Verification items for the finished model (mm, model axes). Coordinates: 2 decimals unless noted, no trailing zeros. Loops run counter-clockwise (first coordinate to the right, second up) from the corner with the lowest first, then second, coordinate; pieces in that order, holes last. Notation, with made-up numbers: (-21.5, 87.25) - (26.5, 87.25) arc R26 cw to (26.5, 125.25) - close; hole circle Ø9 at (-36.75, 78). An arc over 180 degrees is marked (long way). One line per item, written item: value. Start each with the question number.
(1) Draft check along X on faces 1 (the face through (3.95, 2.95, -6.72)), 2 (the face through (-7.794, 3, 0)), 3 (the face through (1.352, 2.958, 4.292)). Enter one of: +X half, -X half, draft (parallel to the pull), parting line (faces both ways), or undercut.
(2) Section check A-A (y = 1.9). Record the boundary of the cut face in (x, z), plus the area to 3 significant figures.
(3) Thickness scan on probe 1 along X at (y, z) = (1.65, 0); probe 2 along X at (y, z) = (4.2, -3); probe 3 along Z at (x, y) = (-0.25, 1). Record the ranges inside material, lowest first. Write a range as [from, to].
(4) Section check C-C (y = 5.4). Record the boundary of the cut face in (x, z), plus the area to 3 significant figures.
(5) Gauge pin test, flat ends, axial feed: P1, Ø7, axis at x = 0, z = 0, coming from the +Y side; P2, Ø2, axis at x = -0.5, y = 1.5, coming from the +Z side; P3, Ø2, axis at x = -3, z = 6, coming from the -Y side; P4, Ø2, axis at x = -1.5, y = 5, coming from the -Z side. Record the tip position at first contact, or that the pin passes through.
```python
from build123d import *

# Parameters (mm, degrees)
SKETCH3_R           = 4.5
BOSS_EXTRUDE2_DEPTH = 6
SKETCH4_OUTSIDE_W   = 42.5
SKETCH4_OUTSIDE_H   = 44.912
SKETCH4_OUTSIDE_R   = 7.768332991
CUT_EXTRUDE1_DEPTH  = 10
CUT_EXTRUDE1_DRAFT  = -45


with BuildPart() as part:
    # Sketch3 → Boss-Extrude2 (new body)
    with BuildSketch(Plane(origin=(0, 0, 0), x_dir=(1, 0, 0), z_dir=(0, 1, 0))):
        Polygon((0, -9), (7.794228634, -4.5), (7.794228634, 4.5), (0, 9), (-7.794228634, 4.5), (-7.794228634, -4.5), align=None)
        with Locations(Location((0, 0, 0), (0, 0, 270))):  # turned: the seam where the file's is
            Circle(SKETCH3_R, mode=Mode.SUBTRACT)
    extrude(amount=BOSS_EXTRUDE2_DEPTH)


with BuildPart() as cut_extrude1_tool:
    # Sketch4 outside → Cut-Extrude1 (with draft: the straight prism first)
    with BuildSketch(Plane(origin=(0, 6, 0), x_dir=(1, 0, 0), z_dir=(0, 1, 0))):
        Rectangle(SKETCH4_OUTSIDE_W, SKETCH4_OUTSIDE_H)
        Circle(SKETCH4_OUTSIDE_R, mode=Mode.SUBTRACT)
    extrude(amount=-CUT_EXTRUDE1_DEPTH)
    # Cut-Extrude1: the draft: its side faces are tilted about the plane it starts from
    cut_extrude1_sides = [cut_extrude1_tool.faces().sort_by_distance(p)[0] for p in [
        (0, 1, 22.456),
        (21.25, 1, 0),
        (0, 1, -22.456),
        (-21.25, 1, 0),
        (-7.768332991, 1, 0),
    ]]
    draft(cut_extrude1_sides, Plane(origin=(0, 6, 0), x_dir=(1, 0, 0), z_dir=(0, 1, 0)), CUT_EXTRUDE1_DRAFT)


with BuildPart() as part_1:
    add(part.part)

    # Cut-Extrude1: cut by cut_extrude1_tool
    add(cut_extrude1_tool.part, mode=Mode.SUBTRACT)


solid = part_1.part
```
Responses:
1. face 1: +X half
1. face 2: -X half
1. face 3: undercut
2. outline: (-7.79, -4.5) - (0, -9) - (7.79, -4.5) - (7.79, 4.5) - (0, 9) - (-7.79, 4.5) - close; hole circle Ø9 at (0, 0)
2. area: 147 mm²
3. probe 1: x = [-7.79, -4.5], [4.5, 7.79]
3. probe 2: x = [-7.79, -3.35], [3.35, 7.79]
3. probe 3: z = [-8.86, -4.49], [4.49, 8.86]
4. outline: (-7.79, -3.05) arc R8.37 ccw to (-6.54, -5.23) - (-1.26, -8.27) arc R8.37 ccw to (1.26, -8.27) - (6.54, -5.23) arc R8.37 ccw to (7.79, -3.05) - (7.79, 3.05) arc R8.37 ccw to (6.54, 5.23) - (1.26, 8.27) arc R8.37 ccw to (-1.26, 8.27) - (-6.54, 5.23) arc R8.37 ccw to (-7.79, 3.05) - close; hole circle Ø9 at (0, 0)
4. area: 142 mm²
5. P1: passes through
5. P2: stops at z = 9
5. P3: stops at y = 0
5. P4: stops at z = -8.71
